Autodesk Fusion 360 part; units mm, degrees
sketch "Sketch2" plane through (0, 0, 0) normal (0, 0, 1) x (1, 0, 0)
  circle A0 centre (0, 0) radius 38.1
  dimension "d15" = 76.2
extrude "Extrude1" add sketch "Sketch2" along normal blind 5
sketch "Sketch3" plane through (0, 0, 5) normal (0, 0, 1) x (-1, 0, 0)
  circle A0 centre (0, 0) radius 38.1
  circle A1 centre (0, 0) radius 19.05
  dimension "d14" = 38.1
extrude "Extrude2" add sketch "Sketch3" along normal blind 22.86 contours A1
sketch "Sketch4" plane through (0, 0, 0) normal (0, 0, -1) x (1, 0, 0)
  circle A0 centre (0, 0) radius 38.1
  circle A1 centre (0.0969, -12.6996) radius 2.2098
  circle A2 centre (10.9498, 6.4337) radius 2.2098
  circle A3 centre (-11.0466, 6.2659) radius 2.2098
  arc A4 (2.2968, -12.4906) -> (11.8992, 4.4383) centre (0, 0) ccw
  arc A5 (9.6688, 8.2343) -> (-9.7933, 8.0859) centre (0, 0) ccw
  arc A6 (-11.9656, 4.2562) -> (-2.106, -12.5242) centre (0, 0) ccw
  dimension "d7" = 4.4196
  dimension "d9" = 360
extrude "Extrude3" add sketch "Sketch4" along normal blind 5 contours A1 | A2 | A3
fillet "Fillet2" radius 8.89 1 edges at (17.7608, 6.8888, 27.86)
fillet "Fillet3" radius 2.54 1 edges at (-35.5217, -13.7775, 5)
Here's how the part is built. I have some questions about the finished solid (model axes, mm). A direction names the side the tool comes from. Coordinates: 2 decimals unless noted, no trailing zeros. Order: outer loops, then holes, each group sorted by start corner. A loop starts at its lowest first (then second) coordinate and runs counter-clockwise, first axis right, second up. Notation, with made-up numbers: (44.5, 84.5) - (102.5, 84.5) arc R27 ccw to (102.5, 112.5) - close; hole circle Ø2 at (-9.75, -40). An arc over 180 degrees is marked (long way). One line per question, with ' | ' between items.
(1) For faces 4 (the cylindrical face through (-30.235, 23.183, 1.213)), 5 (the flat face through (15, -15, 5)), 6 (the cylindrical face through (-11.526, -8.423, -2.465)), which set-ups out of +Z, -Z, +X, -X, +Y, -Y let a thin tool reach every point of the face, with its end or its side?
Report:
face 4: +Z, -Z | face 5: +Z | face 6: -Z
(2) Suppose I cut it at D-D on z = 1.5. List the corners of the cut face in (x, y) for me, and give its area (3 significant figures).
Report:
outline: circle Ø76.2 at (0, 0) | area: 4,560 mm2
(3) If I drill on L1, parallel to Z at x = -19, y = 7; L2, parallel to X at y = 16.5, z = 20; L3, parallel to Y at x = 10, z = 13.5, over which ranges is the centre line in solid material (lowest first)?
Report:
L1: z = 0 to 5 | L2: x = -9.4 to 9.4 | L3: y = -16.21 to 16.21
(4) Suppose I cut it at C-C on z = 23.5. List the corners of the cut face in (x, y) for me, and give its area (3 significant figures).
Report:
outline: circle Ø35.62 at (0, 0) | area: 996 mm2
(5) Suppose I cut it at B-B on x = 0. List the corners of the cut face in (y, z) for me.
Report:
outline: (-38.1, 0) - (10.49, 0) - (10.49, -5) - (14.91, -5) - (14.91, 0) - (38.1, 0) - (38.1, 2.46) arc R2.54 ccw to (35.56, 5) - (19.05, 5) - (19.05, 18.97) arc R8.89 ccw to (10.16, 27.86) - (-10.16, 27.86) arc R8.89 ccw to (-19.05, 18.97) - (-19.05, 5) - (-35.56, 5) arc R2.54 ccw to (-38.1, 2.46) - close
(6) Suppose I cut it at A-A on y = 0. List the corners of the cut face in (x, z) for me.
Report:
outline: (-38.1, 0) - (38.1, 0) - (38.1, 2.46) arc R2.54 ccw to (35.56, 5) - (19.05, 5) - (19.05, 18.97) arc R8.89 ccw to (10.16, 27.86) - (-10.16, 27.86) arc R8.89 ccw to (-19.05, 18.97) - (-19.05, 5) - (-35.56, 5) arc R2.54 ccw to (-38.1, 2.46) - close
(7) Will these pins go through, and if not, where does the flat tip stop? pin 1 (1.5 mm diameter, centred on x = 28, y = -0.5, fed in from -Z); pin 2 (6 mm diameter, centred on x = 6, y = 16.5, fed in from +Z); pin 3 (12 mm diameter, centred on x = 6, z = 12.5, fed in from +Y).
Report:
pin 1: stops at z = 0 | pin 2: stops at z = 26.7 | pin 3: stops at y = 19.05
(8) If we mould it in two halves opening along X, with no side actions, what happens to faces 1 (the cylindrical face through (12.99, -7.28, -2.46)), 2 (the cylindrical face through (-0.38, 10.54, -2.46)), 3 (the flat face through (-11, -6, -5))? For each: pulls with the +X half, pulls with the -X half, needs draft (parallel to the pull), parting line crosses it, or undercut.
Report:
face 1: undercut | face 2: parting line crosses it | face 3: needs draft
